Source: CAD feature listing. Evaluate the final solid. Frame: model axes, mm. Face numbers are marked on the shaded views. Give positions to 0.01 mm unless a question says otherwise; leave off trailing zeros. Loops run counter-clockwise (first coordinate to the right, second up) from the corner with the lowest first, then second, coordinate; pieces in that order, holes last. Notation, with made-up numbers: M 7.25,65 L 46.25,65 A20 ccw 46.25,101 Z; hole C -27.75,64 d4. An arc over 180 degrees is marked long. Answer in a Markdown table with one row per item.
```python
from build123d import *

# Parameters (mm, degrees)
F1_DEPTH = 35
F3_D     = 6
F3_DEPTH = 20
F3_TIP   = 1.8025818571
F5_DEPTH = 35
F7_D     = 2.5
F7_DEPTH = 7.5
F7_TIP   = 0.7510757738


with BuildPart() as f1:
    # F0 (on Front) → F1 (new body)
    with BuildSketch(Plane.XZ):
        Polygon((0, 19.931551069), (0, 0), (35, 0), (35, 19.931551069), (32.5, 19.931551069), (32.5, 21.631551069), (35, 21.631551069), (35, 25.6460141391), (33.5, 25.6460141391), (33.5, 27.1460141391), (35, 27.1460141391), (35, 30.9151932597), (34, 30.9151932597), (34, 31.7151932597), (35, 31.7151932597), (35, 35), (0, 35), (0, 31.7151932597), (1, 31.7151932597), (1, 30.9151932597), (0, 30.9151932597), (0, 27.1460141391), (1.5, 27.1460141391), (1.5, 25.6460141391), (0, 25.6460141391), (0, 21.631551069), (2.5, 21.631551069), (2.5, 19.931551069), align=None)
    extrude(amount=F1_DEPTH)

    # F3
    with Locations(Plane(origin=(0, 0, 0), x_dir=(1, 0, 0), z_dir=(0, 0, -1))):
        with Locations((10, 17.5), (25, 17.5)):
            Hole(F3_D / 2, depth=F3_DEPTH)
            with Locations((0, 0, -(F3_DEPTH + F3_TIP / 2))):  # 118° drill point
                Cone(0, F3_D / 2, F3_TIP, mode=Mode.SUBTRACT)

    # F4 (on face) → F5 (intersect)
    with BuildSketch(Plane.YZ.offset(35)):
        Polygon((-35, 19.931551069), (-35, 0), (0, 0), (0, 19.931551069), (-2.5, 19.931551069), (-2.5, 21.631551069), (0, 21.631551069), (0, 25.6460141391), (-1.5, 25.6460141391), (-1.5, 27.1460141391), (0, 27.1460141391), (0, 30.9151932597), (-1, 30.9151932597), (-1, 31.7151932597), (0, 31.7151932597), (0, 35), (-35, 35), (-35, 31.7151932597), (-34, 31.7151932597), (-34, 30.9151932597), (-35, 30.9151932597), (-35, 27.1460141391), (-33.5, 27.1460141391), (-33.5, 25.6460141391), (-35, 25.6460141391), (-35, 21.631551069), (-32.5, 21.631551069), (-32.5, 19.931551069), align=None)
    extrude(amount=-F5_DEPTH, mode=Mode.INTERSECT)

    # F7
    with Locations(Plane.XY.offset(35)):
        with Locations((30, -30), (30, -5), (5, -5), (5, -30)):
            Hole(F7_D / 2, depth=F7_DEPTH)
            with Locations((0, 0, -(F7_DEPTH + F7_TIP / 2))):  # 118° drill point
                Cone(0, F7_D / 2, F7_TIP, mode=Mode.SUBTRACT)


solid = f1.part
```
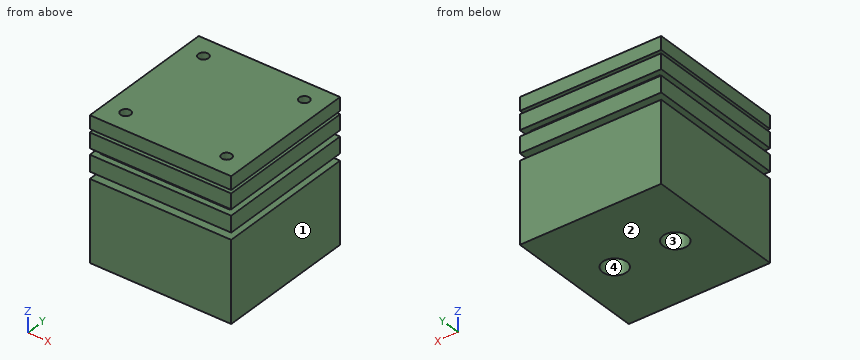
1) Pull-direction query (X, two-part tool) for the marked faces 1, 2, 3 and 4; classes: released by +X, released by -X, zero draft, split by the parting line, or undercut.
Reply:
| item | result |
|---|---|
| face 1 | released by +X |
| face 2 | zero draft |
| face 3 | undercut |
| face 4 | undercut |
2) Section A-A, the plane z = 6. Return loops of the section in (x, y), then the cut area to 3 significant figures.
Reply:
| item | result |
|---|---|
| outline | M 0,-35 L 35,-35 L 35,0 L 0,0 Z; hole C 10,-17.5 d6; hole C 25,-17.5 d6 |
| area | 1,170 mm² |
3) Material intervals for L1, parallel to Y at x = 5, z = 31.5; L2, parallel to Y at x = 5, z = 32.5; L3, parallel to X at y = -5, z = 33, sorted ascending.
Reply:
| item | result |
|---|---|
| L1 | y = -34 to -31.25, -28.75 to -6.25, -3.75 to -1 |
| L2 | y = -35 to -31.25, -28.75 to -6.25, -3.75 to 0 |
| L3 | x = 0 to 3.75, 6.25 to 28.75, 31.25 to 35 |
4) Pin query (flat end, axial travel): pin 1 Ø0.5 at (y, z) = (-25, 20.5) entering from +X. Return the tip coordinate at first contact, or that it passes through.
Reply:
| item | result |
|---|---|
| pin 1 | stops at x = 32.5 |
